For this review, take the finished solid that the model builds, in its own axes (mm). A direction names the side the tool comes from. Round coordinates to 2 decimals unless told otherwise and drop trailing zeros. Order: outer loops, then holes, each group sorted by start corner. A loop starts at its lowest first (then second) coordinate and runs counter-clockwise, first axis right, second up.
from build123d import *

# Parameters (mm, degrees)
SKETCH_1_W          = 100
SKETCH_1_H          = 100
EXTRUDE_1_DEPTH     = 2
SKETCH_2_W          = 2
SKETCH_2_H          = 2
SKETCH_2_W_2        = 38
SKETCH_2_H_2        = 38
EXTRUDE_2_DEPTH     = 20
SKETCH_3_W          = 38
SKETCH_3_H          = 2
SKETCH_3_W_2        = 2
SKETCH_3_H_2        = 38
SKETCH_3_H_3        = 40
SKETCH_3_W_3        = 40
EXTRUDE_3_DEPTH     = 20
RIB_2_REACH         = 133.807
SKETCH_7_WALL_W     = 294.768112702
SKETCH_7_WALL_H     = 2
FILLET_1_R          = 3
RIB_3_REACH         = 133.807
SKETCH_8_WALL_W     = 294.768112702
SKETCH_8_WALL_H     = 2
MIRROR_START        = 20
MIRROR_3_DEPTH      = 2
MIRROR_START_2      = 82
MIRROR_3_2_DEPTH    = 2
MIRROR_START_3      = 2
MIRROR_3_3_DEPTH    = 18
MIRROR_START_4      = 84
MIRROR_3_4_DEPTH    = 14
MIRROR_START_5      = 12
MIRROR_3_5_DEPTH    = 2
SKETCH_10_R         = 2
CUT_EXTRUDE_1_DEPTH = 20
SKETCH_11_R         = 2
CUT_EXTRUDE_2_DEPTH = 20


with BuildPart() as part:
    # 草图1 → 凸台-拉伸1 (new body)
    with BuildSketch(Plane.XY):
        with Locations((50, 50)):
            Rectangle(SKETCH_1_W, SKETCH_1_H)
    extrude(amount=EXTRUDE_1_DEPTH)

    # 草图2 → 凸台-拉伸2 (add)
    with BuildSketch(Plane.XY.offset(2)):
        with Locations((1, 99)):
            Rectangle(SKETCH_2_W, SKETCH_2_H)
        with Locations((21, 99)):
            Rectangle(SKETCH_2_W_2, SKETCH_2_H)
        with Locations((1, 79)):
            Rectangle(SKETCH_2_W, SKETCH_2_H_2)
        with Locations((1, 21)):
            Rectangle(SKETCH_2_W, SKETCH_2_H_2)
        with Locations((1, 1)):
            Rectangle(SKETCH_2_W, SKETCH_2_H)
        with Locations((21, 1)):
            Rectangle(SKETCH_2_W_2, SKETCH_2_H)
    extrude(amount=EXTRUDE_2_DEPTH)

    # 草图3 → 凸台-拉伸3 (add)
    with BuildSketch(Plane.XY.offset(2)):
        with Locations((79, 99)):
            Rectangle(SKETCH_3_W, SKETCH_3_H)
        with Locations((99, 99)):
            Rectangle(SKETCH_3_W_2, SKETCH_3_H)
        with Locations((99, 79)):
            Rectangle(SKETCH_3_W_2, SKETCH_3_H_2)
        with Locations((99, 20)):
            Rectangle(SKETCH_3_W_2, SKETCH_3_H_3)
        with Locations((80, 1)):
            Rectangle(SKETCH_3_W_3, SKETCH_3_H)
    extrude(amount=EXTRUDE_3_DEPTH)

    # 草图7 wall → 筋2 (add, up to next)
    with BuildSketch(Plane(origin=(87.5, 83, 7.5), x_dir=(-0.857492925713, 0, -0.514495755428), z_dir=(0.514495755428, 0, -0.857492925713)), mode=Mode.PRIVATE) as rib_2_sk1:
        Rectangle(SKETCH_7_WALL_W, SKETCH_7_WALL_H)
    rib_2_tool1 = extrude(rib_2_sk1.sketch, amount=RIB_2_REACH, mode=Mode.PRIVATE) - part.part
    rib_2 = rib_2_tool1.solids().sort_by_distance((87.5, 83, 7.5))[0]
    add(rib_2)

    # 圆角1
    fillet_1_edges = [part.edges().sort_by_distance(p)[0] for p in [
        (40, 1, 22),
        (1, 40, 22),
        (1, 60, 22),
        (40, 99, 22),
        (99, 60, 22),
        (60, 99, 22),
        (99, 40, 22),
        (60, 1, 22),
    ]]
    fillet(fillet_1_edges, radius=FILLET_1_R)

    # 草图8 wall → 筋3 (add, up to next)
    with BuildSketch(Plane(origin=(83, 87.5, 7.5), x_dir=(0, 0.857492925713, 0.514495755428), z_dir=(0, 0.514495755428, -0.857492925713)), mode=Mode.PRIVATE) as rib_3_sk1:
        Rectangle(SKETCH_8_WALL_W, SKETCH_8_WALL_H)
    rib_3_tool1 = extrude(rib_3_sk1.sketch, amount=RIB_3_REACH, mode=Mode.PRIVATE) - part.part
    rib_3 = rib_3_tool1.solids().sort_by_distance((83, 87.5, 7.5))[0]
    add(rib_3)

    # 镜向1: 筋3 mirrored; each copy of 筋3 runs up to whatever stops it at its own place
    mirror_1_before = part.part  # the part as the pattern finds it: every copy runs up to it
    mirror_1_rib_3_long = extrude(rib_3_sk1.sketch, amount=RIB_3_REACH, mode=Mode.PRIVATE)
    mirror_1_rib_3_tool1 = mirror_1_rib_3_long.mirror(Plane(origin=(52, 0, 0), x_dir=(0, 0, 1), z_dir=(1, 0, 0))) - mirror_1_before
    add(mirror_1_rib_3_tool1.solids().sort_by_distance((21, 87.5, 7.5))[0])

    # 镜向2: 筋2 mirrored; each copy of 筋2 runs up to whatever stops it at its own place
    mirror_2_before = part.part  # the part as the pattern finds it: every copy runs up to it
    mirror_2_rib_2_long = extrude(rib_2_sk1.sketch, amount=RIB_2_REACH, mode=Mode.PRIVATE)
    mirror_2_rib_2_tool1 = mirror_2_rib_2_long.mirror(Plane(origin=(52, 0, 0), x_dir=(0, 0, 1), z_dir=(1, 0, 0))) - mirror_2_before
    add(mirror_2_rib_2_tool1.solids().sort_by_distance((16.5, 83, 7.5))[0])

    # 镜向3: read off the stored shape, not the designer's step
    # 镜向3 outline → 镜向3 (add)
    with BuildSketch(Plane.YZ.offset(MIRROR_START)):
        Polygon((17.666666667, 2), (14, 4.2), (2, 11.4), (2, 2), align=None)
    extrude(amount=MIRROR_3_DEPTH)

    # Mirror 3 2 outline → Mirror 3 2 (add)
    with BuildSketch(Plane.YZ.offset(MIRROR_START_2)):
        Polygon((14, 2), (14, 4.2), (2, 11.4), (2, 2), align=None)
    extrude(amount=MIRROR_3_2_DEPTH)

    # Mirror 3 3 outline → Mirror 3 3 (add)
    with BuildSketch(Plane.YZ.offset(MIRROR_START_3)):
        Polygon((14, 2), (14, 4.2), (12, 5.4), (12, 2), align=None)
    extrude(amount=MIRROR_3_3_DEPTH)

    # Mirror 3 4 outline → Mirror 3 4 (add)
    with BuildSketch(Plane.YZ.offset(MIRROR_START_4)):
        Polygon((14, 2), (14, 4.2), (12, 5.4), (12, 2), align=None)
    extrude(amount=MIRROR_3_4_DEPTH)

    # Mirror 3 5 outline → Mirror 3 5 (add)
    with BuildSketch(Plane(origin=(0, 0, 0), x_dir=(1, 0, 0), z_dir=(0, 1, 0)).offset(MIRROR_START_5)):
        Polygon((98, -13.8), (98, -2), (78.333333333, -2), align=None)
        Polygon((2, -16.2), (22, -4.2), (20, -4.2), (20, -2), (2, -2), align=None)
    extrude(amount=MIRROR_3_5_DEPTH)

    # 草图10 → 切除-拉伸1 (cut)
    with BuildSketch(Plane.XY.offset(2)):
        with Locations((90, 90)):
            Circle(SKETCH_10_R)
    extrude(amount=-CUT_EXTRUDE_1_DEPTH, mode=Mode.SUBTRACT)

    # 草图11 → 切除-拉伸2 (cut)
    with BuildSketch(Plane.XY.offset(2)):
        with Locations((10, 10)):
            Circle(SKETCH_11_R)
    extrude(amount=-CUT_EXTRUDE_2_DEPTH, mode=Mode.SUBTRACT)


solid = part.part
(1) Wall thickness on L1, parallel to Y at x = 92, z = 5; L2, parallel to Y at x = 25, z = 15: over which ranges is each line inside the solid? List them lowest first.
(2) Add section C-C on y = 72. Give the boundary of the cut face in (x, z), plus the area to 3 significant figures.
(3) Clearance check with flat-ended pins moving along their axes: P1, Ø5, axis at x = 58, y = 21, coming from the +Z side; P2, Ø3, axis at x = 90, y = 90, coming from the -Z side. State where each tip first meets the part, or that it passes through.
(4) Tool access review of faces 1 (the face through (1.01, 39.14, 21.1)), 2 (the face through (11, 91, 2)), 3 (the face through (100, 49, 1)): name each direction out of +Z, -Z, +X, -X, +Y, -Y from which nothing blocks a thin tool from reaching the whole face with its end or side.
(5) Add section A-A on x = 90. Give the boundary of the cut face in (y, z).
(6) Add section B-B on y = 10. Give the boundary of the cut face in (x, z), plus the area to 3 significant figures.
(7) Draft analysis for pull direction Y (two halves, no side actions). For faces 4 (the face through (39.14, 1.01, 21.1)), 5 (the face through (1.01, 60.9, 21.14)), state which applies: pulls with the +Y half, pulls with the -Y half, needs draft (parallel to the pull), parting line crosses it, or undercut.
Here are the results:
1. L1: y = 0 to 2, 12 to 14, 82 to 84, 98 to 100
1. L2: y = 0 to 2, 98 to 100
2. outline: (0, 0) - (100, 0) - (100, 22) - (98, 22) - (98, 2) - (2, 2) - (2, 22) - (0, 22) - close
2. area: 280 mm2
3. P1: stops at z = 2
3. P2: passes through
4. face 1: +Z, +X, -X
4. face 2: +Z
4. face 3: +Z, -Z, +X, +Y, -Y
5. outline: (0, 0) - (88, 0) - (88, 2) - (84, 2) - (84, 9) - (82, 9) - (82, 2) - (14, 2) - (14, 9) - (12, 9) - (12, 2) - (2, 2) - (2, 22) - (0, 22) - close; (92, 0) - (100, 0) - (100, 22) - (98, 22) - (98, 2) - (92, 2) - close
6. outline: (0, 0) - (8, 0) - (8, 2) - (2, 2) - (2, 22) - (0, 22) - close; (12, 0) - (100, 0) - (100, 22) - (98, 22) - (98, 2) - (84, 2) - (84, 6.6) - (82, 6.6) - (82, 2) - (22, 2) - (22, 6.6) - (20, 6.6) - (20, 2) - (12, 2) - close
6. area: 290 mm2
7. face 4: needs draft
7. face 5: undercut
